from build123d import *

# Parameters (mm, degrees)
EXTRUDE_1_DEPTH     = 5
CUT_EXTRUDE_1_DEPTH = 5


with BuildPart() as part:
    # 草图3 → 凸台-拉伸1 (new body)
    with BuildSketch(Plane(origin=(0, 0, 0), x_dir=(0, 0, -1), z_dir=(1, 0, 0))):
        Polygon((-14.574209951, 22.116049871), (1.744837218, 0.483518594), (1.744837218, -19.94046656), (-24.39354953, 14.708582677), align=None)
    extrude(amount=EXTRUDE_1_DEPTH)

    # 草图2 → 切除-拉伸1 (cut)
    with BuildSketch(Plane(origin=(0, 0, 0), x_dir=(0, 0, -1), z_dir=(1, 0, 0))):
        Polygon((-18.40060728, 10.085310763), (-11.774548865, 15.083845536), (-14.966384322, 19.314943078), (-21.592442737, 14.316408305), align=None)
    extrude(amount=CUT_EXTRUDE_1_DEPTH, mode=Mode.SUBTRACT)

    # 镜向1: part across plane


with BuildPart() as part_1:
    add(part.part)
    add(part.part.mirror(Plane(origin=(5, 0.483518594, -1.744837218), x_dir=(1, 0, 0), z_dir=(0, 0, 1))))


solid = part_1.part
Input: part model. Units: mm. Frame: model coordinates. A direction names the side the tool comes from. Give positions to 0.01 mm unless a question says otherwise; leave off trailing zeros. Order: outer loops, then holes, each group sorted by start corner. A loop starts at its lowest first (then second) coordinate and runs counter-clockwise, first axis right, second up. Notation, with made-up numbers: (40, 14.25) - (88, 14.25) arc R38 ccw to (88, 53.25) - close; hole circle Ø7 at (21.25, 51). An arc over 180 degrees is marked (long way). Write each question's results on one line, items separated by ' | '.
Item 1: Section C-C (z = 16). Return loops of the section in (x, y).
A:
outline: (0, 3.58) - (5, 3.58) - (5, 11.9) - (0, 11.9) - close; (0, 18.54) - (5, 18.54) - (5, 21.04) - (0, 21.04) - close
Item 2: Section A-A (x = 3.95). Return loops of the section in (y, z).
A:
outline: (-19.94, -1.74) - (14.71, -27.88) - (22.12, -18.06) - (0.48, -1.74) - (22.12, 14.57) - (14.71, 24.39) - close; hole (10.09, -21.89) - (14.32, -25.08) - (19.31, -18.46) - (15.08, -15.26) - close; hole (10.09, 18.4) - (15.08, 11.77) - (19.31, 14.97) - (14.32, 21.59) - close
Item 3: Section B-B (y = 11). Return loops of the section in (x, z).
A:
outline: (0, -25.09) - (5, -25.09) - (5, -22.58) - (0, -22.58) - close; (0, -20.68) - (5, -20.68) - (5, -9.68) - (0, -9.68) - close; (0, 6.19) - (5, 6.19) - (5, 17.19) - (0, 17.19) - close; (0, 19.09) - (5, 19.09) - (5, 21.6) - (0, 21.6) - close
Item 4: Draft query along Y for faces 1 (the flat face through (2.46, 11.45, -10.02)), 2 (the flat face through (2.46, 12.23, -23.51)), 3 (the flat face through (2.46, -2.86, 11.14)), 4 (the flat face through (5, 1, -7)). Return one class per face: released by +Y, released by -Y, zero draft, split by the parting line, or undercut.
A:
face 1: released by +Y | face 2: undercut | face 3: released by -Y | face 4: zero draft
Item 5: Section D-D (z = -17.5). Return loops of the section in (x, y), and give its area (3 significant figures).
A:
outline: (0, 0.94) - (5, 0.94) - (5, 13.4) - (0, 13.4) - close; (0, 18.05) - (5, 18.05) - (5, 21.37) - (0, 21.37) - close | area: 78.9 mm^2
Item 6: Material intervals for line 1 along Z through (x, y) = (0.2, 13.5); line 2 along Z through (x, y) = (1.55, 17); line 3 along Y through (x, z) = (2.55, -23), sorted ascending.
A:
line 1: z = -26.97 to -24.47, -17.36 to -11.56, 8.07 to 13.87, 20.98 to 23.48 | line 2: z = -24.85 to -21.52, -16.71 to -14.2, 10.71 to 13.22, 18.04 to 21.36 | line 3: y = 8.24 to 11.56, 15.89 to 18.39
Item 7: Contact query for flat-ended pins moving along their axis: pin 1 Ø3 at (x, y) = (2.5, -3.5) entering from -Z; pin 2 Ø1 at (x, z) = (1.5, -4) entering from -Y; pin 3 Ø1 at (x, y) = (3.5, 12) entering from -Z; pin 4 Ø3 at (y, z) = (-2.5, -1) entering from -X. Output: stop coordinate, or through.
A:
pin 1: stops at z = -15.28 | pin 2: stops at y = -17.61 | pin 3: stops at z = -26.22 | pin 4: stops at x = 0
Item 8: Access query for faces 5 (the flat face through (2.46, 11.45, 6.53)), 6 (the flat face through (2.465, 16.851, 18.233)), 7 (the flat face through (2.46, 18.36, 19.55)). Directions: +Z, -Z, +X, -X, +Y, -Y. A direction counts if a zero-diameter tool reaches every point of the face in a straight line with its end or side. Return the directions, or none.
A:
face 5: +X, -X, +Y | face 6: +X, -X | face 7: +Z, +X, -X, +Y
